```python
from build123d import *

# Parameters (mm, degrees)
F0_R     = 1.651
F1_DEPTH = 19.05
F2_R     = 1.651
F3_DEPTH = 19.05
F5_R     = 5.08
F6_R     = 3.302
F7_DEPTH = 12.7
F9_DEPTH = 19.05


with BuildPart() as f1:
    # F0 (on Top) → F1 (new body)
    with BuildSketch(Plane.XY):
        Polygon((9.4747359406, 29.0458423255), (-4.8540289035, -1.3629774042), (2.0390528077, -4.6110267455), (17.0947359406, 27.3404749561), (17.0947359406, 44.8664749561), (9.4747359406, 44.8664749561), align=None)
        Circle(F0_R, mode=Mode.SUBTRACT)
    extrude(amount=F1_DEPTH)

    # F2 (on face) → F3 (cut, through all)
    with BuildSketch(Plane.XY.offset(19.05)):
        Circle(F2_R)
        with Locations((11.811, 26.035)):
            Circle(F2_R)
    extrude(amount=-F3_DEPTH, mode=Mode.SUBTRACT)

    # F5
    f5_edges = [f1.edges().sort_by_distance(p)[0] for p in [
        (9.474736, 44.866475, 9.525),
    ]]
    fillet(f5_edges, radius=F5_R)

    # F6
    f6_edges = [f1.edges().sort_by_distance(p)[0] for p in [
        (-4.854029, -1.362977, 9.525),
        (2.039053, -4.611027, 9.525),
    ]]
    fillet(f6_edges, radius=F6_R)

    # F7 (add): a face of the model
    f7_faces = [f1.faces().sort_by_distance(p)[0] for p in [
        (17.0947359406, 36.1034749561, 9.525),
    ]]
    extrude(f7_faces, amount=F7_DEPTH)

    # F8 (on face) → F9 (join, through all)
    with BuildSketch(Plane.XY.offset(19.05)):
        Polygon((30.3130298853, 0), (29.7947359406, 27.3404749561), (17.0947359406, 27.3404749561), (4.2117881691, 0), align=None)
    extrude(amount=-F9_DEPTH)


solid = f1.part
```
Geometry: final body of the model. Coordinates: model frame, mm. A direction names the side the tool comes from. Coordinates: 2 decimals unless noted, no trailing zeros. Write each loop counter-clockwise with the first axis right and the second up, starting at its lowest first coordinate (ties: lowest second). Pieces come first, ordered by that corner, then holes. Notation, with made-up numbers: M 38,79.25 L 43,79.25 A19 cw 43,111.25 Z; hole C -35,-3 d3. An arc over 180 degrees is marked long. Answer as CSV lines item,"result". Start each with the question number.
Q1. Cut plane D-D on x = 12. Return the cut outline in (y, z), then the cut area to 3 significant figures.
Q2. Mould query, pull axis X, two halves, no side actions, for faces 4 (the flat face through (3.105, 15.527, 9.392)), 5 (the cylindrical face through (1.525, -0.632, 9.392)), 6 (the flat face through (3.824, -0.823, 9.392)). Classes: released by +X, released by -X, zero draft, split by the parting line, or undercut.
Q3. Cut plane B-B on y = 35. Return the cut outline in (x, z), then the cut area to 3 significant figures.
Q4. Reachability of faces 1 (the flat face through (29.795, 36, 9)), 2 (the flat face through (17, 0, 10)), 3 (the flat face through (9.475, 34, 9)) from +Z, -Z, +X, -X, +Y, -Y: full face, straight path, thin tool, end or side. Return the list, or none.
Q5. Line query: line 1 (Y direction, x = 11.5, z = 8.75); line 2 (Y direction, x = -1, z = 17.5); line 3 (X direction, y = 29.5, z = 7.75). Output: solid intervals per line, ascending. Write a range as from..to.
Q6. Cut plane C-C on z = 12. Return the cut outline in (x, y) (3 decimals), then the cut area to 3 significant figures.
Q7. Cut plane A-A on x = 0. Return the cut outline in (y, z).
Q8. Pin query (flat end, axial travel): P1, Ø2, axis at x = 17, y = 17.5, coming from the -Z side; P2, Ø2, axis at x = 5, z = 10, coming from the -Y side; P3, Ø6, axis at x = 10.5, z = 16, coming from the +Y side; P4, Ø5.5, axis at y = 34, z = 8.5, coming from the -X side. Return the tip coordinate at first contact, or that it passes through.
Findings below:
1,outline,"M 0,0 L 24.39,0 L 24.39,19.05 L 0,19.05 Z; M 27.68,0 L 44.18,0 L 44.18,19.05 L 27.68,19.05 Z"
1,area,"779 mm2"
2,face 4,"released by -X"
2,face 5,"undercut"
2,face 6,"released by +X"
3,outline,"M 9.47,0 L 29.79,0 L 29.79,19.05 L 9.47,19.05 Z"
3,area,"387 mm2"
4,face 1,"+Z, -Z, +X, +Y"
4,face 2,"+Z, -Z, +X, -Y"
4,face 3,"+Z, -Z, -X, +Y"
5,line 1,"y = 0..24.41, 27.66..43.85"
5,line 2,"y = -3.18..-1.31, 1.31..6.82"
5,line 3,"x = 9.47..29.79"
6,outline,"M -3.447,1.624 A3.302 ccw -1.867,-2.77 L -0.948,-3.204 A3.302 ccw 3.447,-1.624 L 4.212,0 L 30.313,0 L 29.795,27.34 L 29.795,44.866 L 14.555,44.866 A5.08 ccw 9.475,39.786 L 9.475,29.046 Z; hole C 0,0 d3.302; hole C 11.811,26.035 d3.302"
6,area,"1,120 mm2"
7,outline,"M -3.49,0 L -1.65,0 L -1.65,19.05 L -3.49,19.05 Z; M 1.65,0 L 8.94,0 L 8.94,19.05 L 1.65,19.05 Z"
8,P1,"stops at z = 0"
8,P2,"stops at y = -0.45"
8,P3,"stops at y = 44.76"
8,P4,"stops at x = 9.47"
